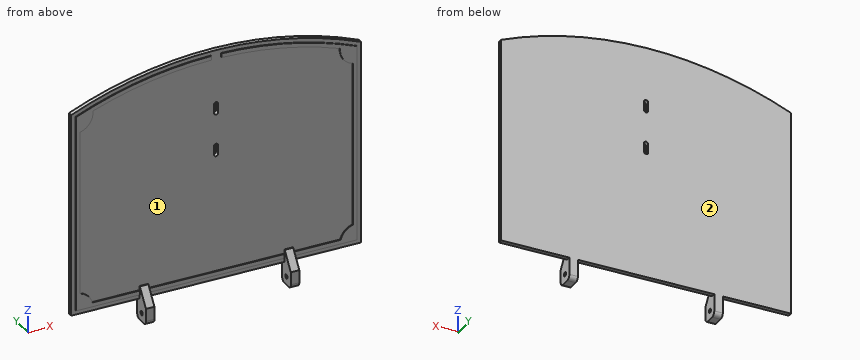
from build123d import *

# Parameters (mm, degrees)
F0_W       = 10
F0_H       = 15
F1_DEPTH   = 5
F3_DEPTH   = 1
F0_H_2     = 25
F4_DEPTH   = 20
F5_SIZE2   = 20
F5_SIZE    = 14
F5_2_SIZE2 = 20
F5_2_SIZE  = 14
F6_R       = 5
F8_D       = 5
F10_DEPTH  = 5


# Not quite as in the source:
# - a feature names something its author has since deleted; it is built from what else it names


with BuildPart() as f1:
    # F0 (on Front) → F1 (new body)
    with BuildSketch(Plane.XZ):
        with BuildLine():
            ThreePointArc((170, 128.3675199291), (0, 162.5), (-170, 128.3675199291))
            Line((-170, 128.3675199291), (-170, -112.5))
            Line((-170, -112.5), (-90, -112.5))
            Line((-90, -112.5), (-90, -97.5))
            Line((-90, -97.5), (-80, -97.5))
            Line((-80, -97.5), (-80, -112.5))
            Line((-80, -112.5), (80, -112.5))
            Line((80, -112.5), (80, -97.5))
            Line((80, -97.5), (90, -97.5))
            Line((90, -97.5), (90, -112.5))
            Line((90, -112.5), (170, -112.5))
            Line((170, -112.5), (170, 128.3675199291))
        make_face()
        with Locations((-85, -105)):
            Rectangle(F0_W, F0_H)
        with Locations((85, -105)):
            Rectangle(F0_W, F0_H)
    extrude(amount=F1_DEPTH)

    # F2 (on face) → F3 (join)
    with BuildSketch(Plane.XZ.offset(5)):
        with BuildLine():
            ThreePointArc((-6, 157.4586583244), (-87.0242594123, 148.7148510214), (-165, 125.0258523247))
            Line((-165, 125.0258523247), (-165, -107.5))
            Line((-165, -107.5), (165, -107.5))
            Line((165, -107.5), (165, 125.0258523247))
            ThreePointArc((165, 125.0258523247), (87.0242594123, 148.7148510214), (6, 157.4586583244))
            Line((6, 157.4586583244), (6, 152.4581780262))
            ThreePointArc((6, 152.4581780262), (76.6048494822, 145.628140857), (145.1290810133, 127.294459524))
            ThreePointArc((145.1290810133, 127.294459524), (148.5184044395, 113.696377148), (160, 105.6609355937))
            Line((160, 105.6609355937), (160, -88.135083269))
            ThreePointArc((160, -88.135083269), (150.8578643763, -93.3578643763), (145.635083269, -102.5))
            Line((145.635083269, -102.5), (-145.635083269, -102.5))
            ThreePointArc((-145.635083269, -102.5), (-150.8578643763, -93.3578643763), (-160, -88.135083269))
            Line((-160, -88.135083269), (-160, 105.6609355937))
            ThreePointArc((-160, 105.6609355937), (-148.5184044395, 113.696377148), (-145.1290810133, 127.294459524))
            ThreePointArc((-145.1290810133, 127.294459524), (-76.6048494822, 145.628140857), (-6, 152.4581780262))
            Line((-6, 152.4581780262), (-6, 157.4586583244))
        make_face()
    extrude(amount=F3_DEPTH)

    # F0 (on Front) → F4 (join)
    with BuildSketch(Plane.XZ):
        with Locations((-85, -125)):
            Rectangle(F0_W, F0_H_2)
        with Locations((85, -125)):
            Rectangle(F0_W, F0_H_2)
        with Locations((85, -105)):
            Rectangle(F0_W, F0_H)
        with Locations((-85, -105)):
            Rectangle(F0_W, F0_H)
    extrude(amount=F4_DEPTH)

    # F5
    f5_edges = [f1.edges().sort_by_distance(p)[0] for p in [
        (85, -20, -97.5),
    ]]
    f5_side = f1.faces().sort_by_distance((85, -12.5, -97.5))[0]
    chamfer(f5_edges, length=F5_SIZE, length2=F5_SIZE2, reference=f5_side)

    # F5#2
    f5_2_edges = [f1.edges().sort_by_distance(p)[0] for p in [
        (-85, -20, -97.5),
    ]]
    f5_2_side = f1.faces().sort_by_distance((-85, -12.5, -97.5))[0]
    chamfer(f5_2_edges, length=F5_2_SIZE, length2=F5_2_SIZE2, reference=f5_2_side)

    # F6
    f6_edges = [f1.edges().sort_by_distance(p)[0] for p in [
        (-85, -20, -137.5),
        (85, -20, -137.5),
        (-85, 0, -137.5),
        (85, 0, -137.5),
    ]]
    fillet(f6_edges, radius=F6_R)

    # F8 (through all)
    with Locations(Plane.YZ.offset(90)):
        with Locations((-10, -127.5)):
            Hole(F8_D / 2)

    # F9 (on face) → F10 (cut)
    with BuildSketch(Plane.XZ.offset(5)):
        with BuildLine():
            Line((2.5, 87.5), (2.5, 97.5))
            ThreePointArc((2.5, 97.5), (0, 100), (-2.5, 97.5))
            Line((-2.5, 97.5), (-2.5, 87.5))
            ThreePointArc((-2.5, 87.5), (0, 85), (2.5, 87.5))
        make_face()
        with BuildLine():
            Line((2.5, 37.5), (2.5, 47.5))
            ThreePointArc((2.5, 47.5), (0, 50), (-2.5, 47.5))
            Line((-2.5, 47.5), (-2.5, 37.5))
            ThreePointArc((-2.5, 37.5), (0, 35), (2.5, 37.5))
        make_face()
    extrude(amount=-F10_DEPTH, mode=Mode.SUBTRACT)


solid = f1.part
Input: part model. Units: mm. Frame: model coordinates. Face numbers are marked on the shaded views. Round coordinates to 2 decimals unless told otherwise and drop trailing zeros. Loops run counter-clockwise (first coordinate to the right, second up) from the corner with the lowest first, then second, coordinate; pieces in that order, holes last. Notation, with made-up numbers: M -18,48.25 L 10,48.25 A28 cw 10,79.25 Z; hole C 50,-25 d10. An arc over 180 degrees is marked long. Answer as CSV lines item,"result". Start each with the question number.
(1) Line query: line 1 (X direction, y = -4.5, z = -117.5); line 2 (Y direction, x = -83, z = -127); line 3 (X direction, y = -5.75, z = -78.5). Output: solid intervals per line, ascending. Write a range as [from, to].
(2) Section A-A, the plane z = -15. Output: boundary loops of the cut face in (x, y), plus the area to 3 significant figures.
(3) Draft query along X for the marked faces 1 and 2. Return one class per face: released by +X, released by -X, zero draft, split by the parting line, or undercut.
(4) Section C-C, the plane x = -57. Output: boundary loops of the cut face in (y, z), plus the area to 3 significant figures.
(5) Section B-B, the plane x = 86. Output: boundary loops of the cut face in (y, z), plus the area to 3 significant figures.
(6) First-contact query: pin 1 (3 mm diameter, centred on y = -10, z = -127.5, fed in from -X); pin 2 (1.5 mm diameter, centred on x = -7.5, z = -104.5, fed in from -Y); pin 3 (2.5 mm diameter, centred on x = -5.5, z = -109.5, fed in from -Y); pin 4 (4 mm diameter, centred on x = -13, y = -2, fed in from -Z). Flat tips, straight axial feed; report the tip coordinate or a pass-through.
Values found:
1,line 1,"x = [-90, -80], [80, 90]"
1,line 2,"y = [-20, -12.45], [-7.55, 0]"
1,line 3,"x = [-165, -160], [160, 165]"
2,outline,"M -170,-5 L -165,-5 L -165,-6 L -160,-6 L -160,-5 L 160,-5 L 160,-6 L 165,-6 L 165,-5 L 170,-5 L 170,0 L -170,0 Z"
2,area,"1,710 mm²"
3,face 1,"undercut"
3,face 2,"zero draft"
4,outline,"M -6,-107.5 L -5,-107.5 L -5,-112.5 L 0,-112.5 L 0,158.8 L -5,158.8 L -5,153.75 L -6,153.75 L -6,148.71 L -5,148.71 L -5,-102.5 L -6,-102.5 Z"
4,area,"1,370 mm²"
5,outline,"M -20,-132.5 A5 ccw -15,-137.5 L -5,-137.5 A5 ccw 0,-132.5 L 0,154.02 L -5,154.02 L -5,148.92 L -6,148.92 L -6,143.82 L -5,143.82 L -5,-97.5 L -6,-97.5 L -20,-117.5 Z; hole C -10,-127.5 d5"
5,area,"1,890 mm²"
6,pin 1,"passes through"
6,pin 2,"stops at y = -6"
6,pin 3,"stops at y = -5"
6,pin 4,"stops at z = -112.5"
